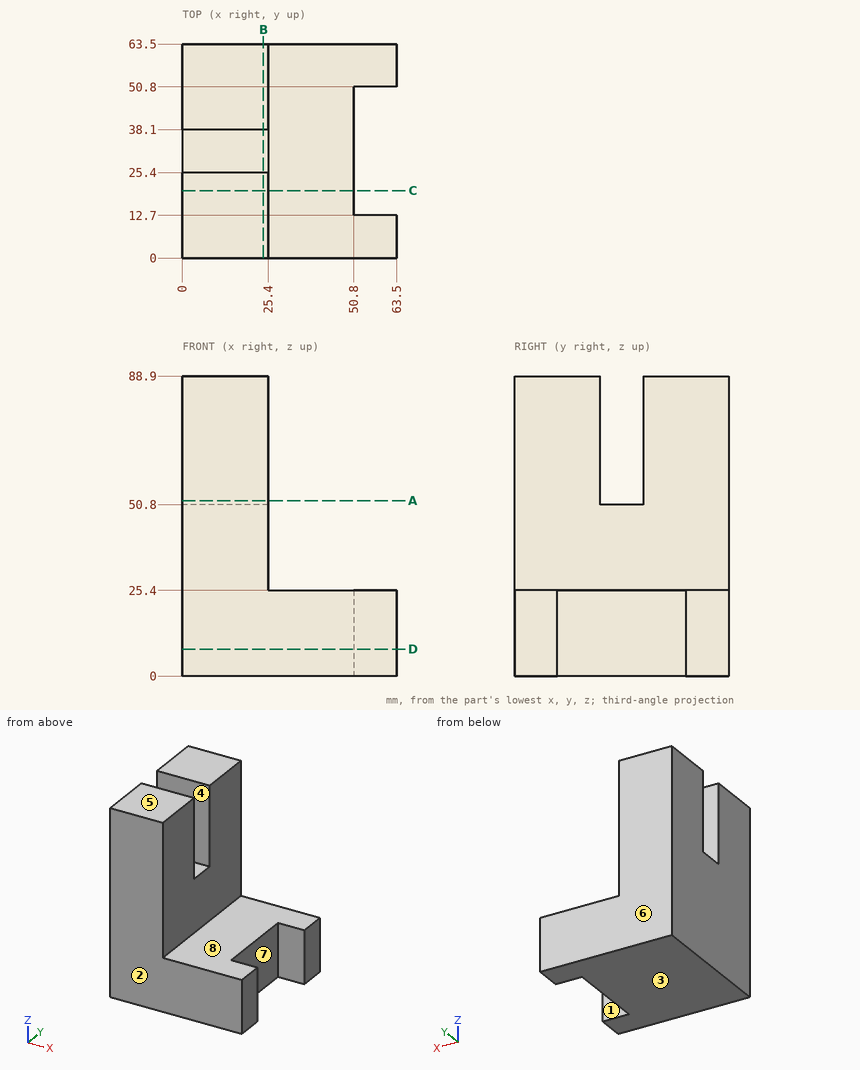
Input: dimensioned drawing with shaded views. Units: mm. Origin: part minimum x, y, z. A direction names the side the tool comes from. Coordinates: 2 decimals unless noted, no trailing zeros. Write each loop counter-clockwise with the first axis right and the second up, starting at its lowest first coordinate (ties: lowest second). Pieces come first, ordered by that corner, then holes. Notation, with made-up numbers: (56, 32) -> (82, 32) arc R23 cw to (82, 48) -> close; hole circle Ø6 at (-12.5, 15). An arc over 180 degrees is marked (long way). Return JSON: item names as keys, results as strings. Group by question number.
1) Section query D-D, the plane z = 8. Return loops of the section in (x, y).
2) Ray query, line 1 along Y through (x, z) = (9.5, 83.5); line 2 along Z through (x, y) = (50, 57); line 3 along X through (y, z) = (47.5, 17.5). Return the intervals inside material, ascending.
3) Section query C-C, the plane y = 20. Return loops of the section in (x, z).
4) Mould query, pull axis Y, two halves, no side actions, for the marked faces 1, 2 and 3. Classes: +Y half, -Y half, draft (parallel to the pull), parting line (faces both ways), or undercut.
5) Set-up query: the marked faces 4, 5, 6, 7 and 8. Return all of +Z, -Z, +X, -X, +Y, -Y with unobstructed straight access to the full face (end or side cutting, diameter ignored); none if empty.
6) Section query B-B, the plane x = 24. Return loops of the section in (y, z), plus the area to 3 significant figures.
7) Section query A-A, the plane z = 52. Return loops of the section in (x, y), plus the area to 3 significant figures.
8) Contact query for flat-ended pins moving along their axis: P1, Ø12, axis at y = 48.5, z = 53, coming from the +X side; P2, Ø8, axis at x = 39, y = 7.5, coming from the +Z side; P3, Ø6.5, axis at x = 16, y = 32, coming from the +Z side. Output: stop coordinate, or through.
From the geometry:
{
 "1": {"outline": "(0, 0) -> (63.5, 0) -> (63.5, 12.7) -> (50.8, 12.7) -> (50.8, 50.8) -> (63.5, 50.8) -> (63.5, 63.5) -> (0, 63.5) -> close"},
 "2": {"line 1": "0 to 25.4, 38.1 to 63.5", "line 2": "0 to 25.4", "line 3": "0 to 50.8"},
 "3": {"outline": "(0, 0) -> (50.8, 0) -> (50.8, 25.4) -> (25.4, 25.4) -> (25.4, 88.9) -> (0, 88.9) -> close"},
 "4": {"face 1": "undercut", "face 2": "-Y half", "face 3": "draft"},
 "5": {"face 4": "+Z, +X, -X", "face 5": "+Z, +X, -X, +Y, -Y", "face 6": "+Z, -Z, +X, -X, +Y", "face 7": "+Z, -Z, +X", "face 8": "+Z, +X, +Y, -Y"},
 "6": {"outline": "(0, 0) -> (63.5, 0) -> (63.5, 88.9) -> (38.1, 88.9) -> (38.1, 50.8) -> (25.4, 50.8) -> (25.4, 88.9) -> (0, 88.9) -> close", "area": "5,160 mm²"},
 "7": {"outline": "(0, 0) -> (25.4, 0) -> (25.4, 25.4) -> (0, 25.4) -> close; (0, 38.1) -> (25.4, 38.1) -> (25.4, 63.5) -> (0, 63.5) -> close", "area": "1,290 mm²"},
 "8": {"P1": "x = 25.4", "P2": "z = 25.4", "P3": "z = 50.8"}
}
